from build123d import *

# Parameters (mm, degrees)
SKETCH_W     = 52
SKETCH_H     = 66
SKETCH_R     = 1.6
SKETCH_R_2   = 1
PAD_DEPTH    = 3
FILLET_R     = 2
SKETCH001_W  = 40
SKETCH001_H  = 45
POCKET_DEPTH = 5
FILLET001_R  = 5


with BuildPart() as part:
    # Sketch → Pad (new body)
    with BuildSketch(Plane.XY):
        Rectangle(SKETCH_W, SKETCH_H)
        with Locations((-22.5, 29)):
            Circle(SKETCH_R, mode=Mode.SUBTRACT)
        with Locations((-9, 29)):
            Circle(SKETCH_R_2, mode=Mode.SUBTRACT)
        with Locations((-3, 29)):
            Circle(SKETCH_R_2, mode=Mode.SUBTRACT)
        with Locations((3, 29)):
            Circle(SKETCH_R_2, mode=Mode.SUBTRACT)
        with Locations((9, 29)):
            Circle(SKETCH_R_2, mode=Mode.SUBTRACT)
        with Locations((22.5, 29)):
            Circle(SKETCH_R, mode=Mode.SUBTRACT)
        with Locations((-22.5, -29)):
            Circle(SKETCH_R, mode=Mode.SUBTRACT)
        with Locations((-9, -29)):
            Circle(SKETCH_R_2, mode=Mode.SUBTRACT)
        with Locations((-3, -29)):
            Circle(SKETCH_R_2, mode=Mode.SUBTRACT)
        with Locations((3, -29)):
            Circle(SKETCH_R_2, mode=Mode.SUBTRACT)
        with Locations((9, -29)):
            Circle(SKETCH_R_2, mode=Mode.SUBTRACT)
        with Locations((22.5, -29)):
            Circle(SKETCH_R, mode=Mode.SUBTRACT)
    extrude(amount=PAD_DEPTH)

    # Fillet
    fillet_edges = [part.edges().sort_by_distance(p)[0] for p in [
        (26, -33, 1.5),
        (-26, -33, 1.5),
        (26, 33, 1.5),
        (-26, 33, 1.5),
    ]]
    fillet(fillet_edges, radius=FILLET_R)

    # Sketch001 (on Face5 of Fillet) → Pocket (cut)
    with BuildSketch(Plane.XY.offset(3)):
        Rectangle(SKETCH001_W, SKETCH001_H)
    extrude(amount=-POCKET_DEPTH, mode=Mode.SUBTRACT)

    # Fillet001
    fillet001_edges = [part.edges().sort_by_distance(p)[0] for p in [
        (20, -22.5, 1.5),
        (-20, 22.5, 1.5),
        (20, 22.5, 1.5),
        (-20, -22.5, 1.5),
    ]]
    fillet(fillet001_edges, radius=FILLET001_R)


solid = part.part
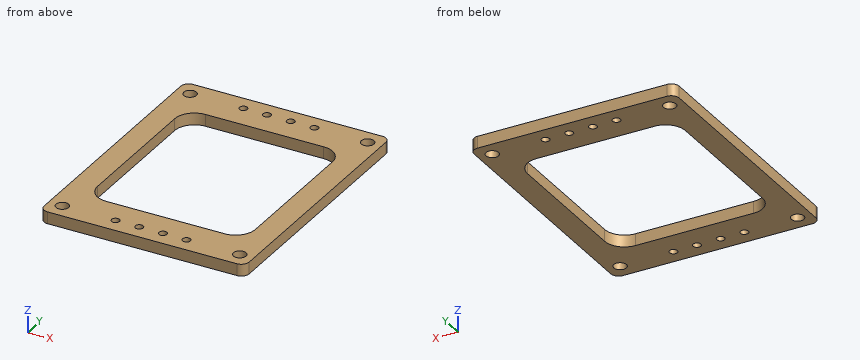
Geometry: final body of the model. Coordinates: model frame, mm. Give positions to 0.01 mm unless a question says otherwise; leave off trailing zeros. Loops run counter-clockwise (first coordinate to the right, second up) from the corner with the lowest first, then second, coordinate; pieces in that order, holes last. Notation, with made-up numbers: M 10,23.25 L 31,23.25 A25 cw 31,49.25 Z; hole C 77,47 d6. An arc over 180 degrees is marked long. Put each result on its own line as item: value. Start each with the question number.
1) Cut plane C-C (z = 0.75). Give the number of separate pieces and of enclosed holes in the cut face, then the cut area to 3 significant figures.
2) Cut plane D-D (x = 7). Output: boundary loops of the cut face in (y, z).
3) Ray query, line 1 along Y through (x, z) = (22.5, 1.55); line 2 along Y through (x, z) = (-9, 0.9); line 3 along X through (y, z) = (-14, 1.3). Return the intervals inside material, ascending.
4) Cut plane B-B (x = -22.5). Output: boundary loops of the cut face in (y, z).
5) Contact query for a flat-ended pin moving along its axis: pin 1 (1.6 mm diameter, centred on x = 9, y = 29, fed in from +Z). Output: stop coordinate, or through.
6) Cut plane A-A (y = 13). Output: boundary loops of the cut face in (x, z), then the cut area to 3 significant figures.
Verdict:
1. separate pieces: 1
1. enclosed holes: 13
1. area: 1,590 mm2
2. outline: M -33,0 L -22.5,0 L -22.5,3 L -33,3 Z; M 22.5,0 L 33,0 L 33,3 L 22.5,3 Z
3. line 1: -33 to -30.6, -27.4 to 27.4, 30.6 to 33
3. line 2: -33 to -30, -28 to -22.5, 22.5 to 28, 30 to 33
3. line 3: -26 to -20, 20 to 26
4. outline: M -33,0 L -30.6,0 L -30.6,3 L -33,3 Z; M -27.4,0 L 27.4,0 L 27.4,3 L -27.4,3 Z; M 30.6,0 L 33,0 L 33,3 L 30.6,3 Z
5. pin 1: through
6. outline: M -26,0 L -20,0 L -20,3 L -26,3 Z; M 20,0 L 26,0 L 26,3 L 20,3 Z
6. area: 36.0 mm2
